Design review of the part built by this model. Coordinates are the model's own, in mm. A direction names the side the tool comes from. Round coordinates to 2 decimals unless told otherwise and drop trailing zeros. Loops run counter-clockwise (first coordinate to the right, second up) from the corner with the lowest first, then second, coordinate; pieces in that order, holes last. Notation, with made-up numbers: (41, 17) - (82, 17) arc R16 cw to (82, 35) - close; hole circle Ø2 at (-15, -40). An arc over 180 degrees is marked (long way). Return JSON: item names as keys, results as strings. Group by question number.
(1) The part is to be moulded in two halves that separate along X. For faces 3 (the flat face through (0, 65, 5)), 4 (the cylindrical face through (32.027, -40.641, 4.93)), 5 (the cylindrical face through (38, 64, 5)), say which applies: pulls with the +X half, pulls with the -X half, needs draft (parallel to the pull), parting line crosses it, or undercut.
(2) Clearance check with a flat-ended pin moving along its axis: pin 1 (5 mm diameter, centred on x = 8.34, y = -25.68, fed in from +Z). State where the tip first meets the part, or that it passes through.
(3) Wall thickness on L1, parallel to Y at x = 27.5, z = 2; L2, parallel to X at y = -54, z = 8; L3, parallel to X at y = 9.5, z = 1.5: over which ranges is each line inside the solid? List them lowest first. Write a range as [from, to].
(4) We need section C-C, the plane z = 5.25. Give the number of separate pieces and of enclosed holes in the cut face, and give its area (3 significant figures).
(5) We need section B-B, the plane y = 0. Write out the cut boundary in (x, z), and give its area (3 significant figures).
(6) For faces 1 (the cylindrical face through (-0.705, 23.827, 8.521)), 2 (the cylindrical face through (-27.973, 44.359, 4.93)), list the 3-axis set-ups (+Z, -Z, +X, -X, +Y, -Y) from which the entire face can be reached by the end or side of a thin tool; tool diameter is ignored.
(7) We need section A-A, the plane y = 42.5. Write out the cut boundary in (x, z).
from build123d import *

# Parameters (mm, degrees)
SKETCH1_W                                           = 80
SKETCH1_H                                           = 130
SKETCH1_R                                           = 22.5
BOSS_EXTRUDE1_DEPTH                                 = 10
CBORE_FOR_M3_HEX_SOCKET_HEAD_CAP_SCREW1_D           = 3.5
CBORE_FOR_M3_HEX_SOCKET_HEAD_CAP_SCREW1_CBORE_D     = 6.5
CBORE_FOR_M3_HEX_SOCKET_HEAD_CAP_SCREW1_CBORE_DEPTH = 3
CHAMFER1_SIZE                                       = 1
F_5_5_5_5_DIAMETER_HOLE1_D                          = 5.5
FILLET1_R                                           = 5
M3_TAPPED_HOLE1_D                                   = 2.5


with BuildPart() as part:
    # Sketch1 → Boss-Extrude1 (new body)
    with BuildSketch(Plane.XY):
        Rectangle(SKETCH1_W, SKETCH1_H)
        Circle(SKETCH1_R, mode=Mode.SUBTRACT)
    extrude(amount=BOSS_EXTRUDE1_DEPTH)

    # CBORE for M3 Hex Socket Head Cap Screw1 (through all)
    with Locations(Plane.XY.offset(10)):
        with Locations((-27, 0), (-25.67852594, -8.343458848), (-21.843458848, -15.870201812), (-15.870201812, -21.843458848), (27, 0), (25.67852594, 8.343458848), (21.843458848, 15.870201812), (15.870201812, 21.843458848), (0, 27), (-8.343458848, 25.67852594), (-15.870201812, 21.843458848), (-21.843458848, 15.870201812), (0, -27), (8.343458848, -25.67852594), (15.870201812, -21.843458848), (21.843458848, -15.870201812)):
            CounterBoreHole(CBORE_FOR_M3_HEX_SOCKET_HEAD_CAP_SCREW1_D / 2, CBORE_FOR_M3_HEX_SOCKET_HEAD_CAP_SCREW1_CBORE_D / 2, CBORE_FOR_M3_HEX_SOCKET_HEAD_CAP_SCREW1_CBORE_DEPTH)

    # Chamfer1
    chamfer1_edges = [part.edges().sort_by_distance(p)[0] for p in [
        (-22.5, 0, 0),
    ]]
    chamfer(chamfer1_edges, length=CHAMFER1_SIZE)

    # Ø5.5 (5.5) Diameter Hole1 (through all)
    with Locations(Plane.XY.offset(10)):
        with Locations((-30, 57.5), (30, 57.5), (30, -57.5), (-30, -57.5), (-30, -42.5), (-30, 42.5), (30, 42.5), (30, -42.5)):
            Hole(F_5_5_5_5_DIAMETER_HOLE1_D / 2)

    # Fillet1
    fillet1_edges = [part.edges().sort_by_distance(p)[0] for p in [
        (-40, 65, 5),
        (40, 65, 5),
        (40, -65, 5),
        (-40, -65, 5),
    ]]
    fillet(fillet1_edges, radius=FILLET1_R)

    # M3 Tapped Hole1 (through all)
    with Locations(Plane(origin=(0, 0, 0), x_dir=(-1, 0, 0), z_dir=(0, 0, -1))):
        with Locations((-7.5, -55), (7.5, -55)):
            Hole(M3_TAPPED_HOLE1_D / 2)


solid = part.part
Solutions:
{
 "1": {"face 3": "needs draft", "face 4": "undercut", "face 5": "pulls with the +X half"},
 "2": {"pin 1": "z = 7"},
 "3": {"L1": "[-65, -58.65], [-56.35, -43.65], [-41.35, -1.68], [1.68, 41.35], [43.65, 56.35], [58.65, 65]", "L2": "[-40, -8.25], [-6.75, 6.75], [8.25, 40]", "L3": "[-40, -20.4], [20.4, 24.37], [26.99, 40]"},
 "4": {"separate pieces": "1", "enclosed holes": "27", "area": "8,430 mm^2"},
 "5": {"outline": "(-40, 0) - (-28.75, 0) - (-28.75, 7) - (-30.25, 7) - (-30.25, 10) - (-40, 10) - close; (-25.25, 0) - (-23.5, 0) - (-22.5, 1) - (-22.5, 10) - (-23.75, 10) - (-23.75, 7) - (-25.25, 7) - close; (22.5, 1) - (23.5, 0) - (25.25, 0) - (25.25, 7) - (23.75, 7) - (23.75, 10) - (22.5, 10) - close; (28.75, 0) - (40, 0) - (40, 10) - (30.25, 10) - (30.25, 7) - (28.75, 7) - close", "area": "261 mm^2"},
 "6": {"face 1": "+Z", "face 2": "+Z, -Z"},
 "7": {"outline": "(-40, 0) - (-32.75, 0) - (-32.75, 10) - (-40, 10) - close; (-27.25, 0) - (27.25, 0) - (27.25, 10) - (-27.25, 10) - close; (32.75, 0) - (40, 0) - (40, 10) - (32.75, 10) - close"}
}
